For this review, take the finished solid that the model builds, in its own axes (mm). Coordinates: 2 decimals unless noted, no trailing zeros. Order: outer loops, then holes, each group sorted by start corner. A loop starts at its lowest first (then second) coordinate and runs counter-clockwise, first axis right, second up.
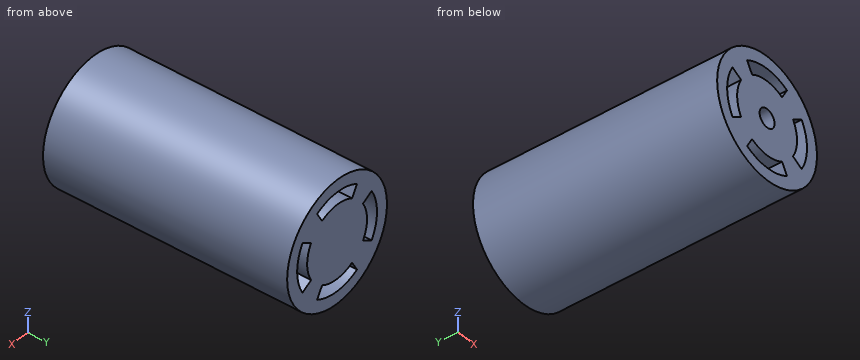
from build123d import *

# Parameters (mm, degrees)
SKETCH1_R           = 5
BOSS_EXTRUDE1_DEPTH = 20
SKETCH2_R           = 0.75
CUT_EXTRUDE1_DEPTH  = 15


with BuildPart() as part:
    # Sketch1 → Boss-Extrude1 (new body)
    with BuildSketch(Plane(origin=(0, 0, 0), x_dir=(1, 0, 0), z_dir=(0, 1, 0))):
        with Locations(Location((0, 0, 0), (0, 0, 270))):
            Circle(SKETCH1_R)
        with BuildLine():
            Line((-2, 3.464101615), (-1.5, 2.598076211))
            ThreePointArc((-1.5, 2.598076211), (0, 3), (1.5, 2.598076211))
            Line((1.5, 2.598076211), (2, 3.464101615))
            ThreePointArc((2, 3.464101615), (0, 4), (-2, 3.464101615))
        make_face(mode=Mode.SUBTRACT)
        with BuildLine():
            Line((2.598076211, -1.5), (3.464101615, -2))
            ThreePointArc((3.464101615, -2), (4, 0), (3.464101615, 2))
            Line((3.464101615, 2), (2.598076211, 1.5))
            ThreePointArc((2.598076211, 1.5), (3, 0), (2.598076211, -1.5))
        make_face(mode=Mode.SUBTRACT)
        with BuildLine():
            Line((-1.5, -2.598076211), (-2, -3.464101615))
            ThreePointArc((-2, -3.464101615), (0, -4), (2, -3.464101615))
            Line((2, -3.464101615), (1.5, -2.598076211))
            ThreePointArc((1.5, -2.598076211), (0, -3), (-1.5, -2.598076211))
        make_face(mode=Mode.SUBTRACT)
        with BuildLine():
            Line((-2.598076211, 1.5), (-3.464101615, 2))
            ThreePointArc((-3.464101615, 2), (-4, 0), (-3.464101615, -2))
            Line((-3.464101615, -2), (-2.598076211, -1.5))
            ThreePointArc((-2.598076211, -1.5), (-3, 0), (-2.598076211, 1.5))
        make_face(mode=Mode.SUBTRACT)
    extrude(amount=BOSS_EXTRUDE1_DEPTH)

    # Sketch2 → Cut-Extrude1 (cut)
    with BuildSketch(Plane.XZ):
        with Locations(Location((0, 0, 0), (0, 0, 270))):
            Circle(SKETCH2_R)
    extrude(amount=-CUT_EXTRUDE1_DEPTH, mode=Mode.SUBTRACT)


solid = part.part
1. Take a section at A-A, the plane x = 0. Give the boundary of the cut face in (y, z), plus the area to 4 significant figures.
Answer below:
outline: (0, -5) - (20, -5) - (20, -4) - (0, -4) - close; (0, -3) - (20, -3) - (20, 3) - (0, 3) - (0, 0.75) - (15, 0.75) - (15, -0.75) - (0, -0.75) - close; (0, 4) - (20, 4) - (20, 5) - (0, 5) - close
area: 137.5 mm2
2. To check wall thickness, follow L1, parallel to X at y = 5.25, z = 0; L2, parallel to X at y = 1.5, z = -2.75; L3, parallel to Z at x = -1.75, y = 18. State the ranges of each line that lie inside material, in increasing order.
Answer below:
L1: x = -5 to -4, -3 to -0.75, 0.75 to 3, 4 to 5
L2: x = -4.18 to -1.59, -1.2 to 1.2, 1.59 to 4.18
L3: z = -4.68 to -3.6, -3.03 to 3.03, 3.6 to 4.68
3. Take a section at D-D, the plane y = 18. Give the boundary of the cut face in (x, z).
Answer below:
outline: circle Ø10 at (0, 0); hole (-3.46, -2) - (-2.6, -1.5) arc R3 cw to (-2.6, 1.5) - (-3.46, 2) arc R4 ccw to start; hole (-2, -3.46) arc R4 ccw to (2, -3.46) - (1.5, -2.6) arc R3 cw to (-1.5, -2.6) - close; hole (-2, 3.46) - (-1.5, 2.6) arc R3 cw to (1.5, 2.6) - (2, 3.46) arc R4 ccw to start; hole (2.6, -1.5) - (3.46, -2) arc R4 ccw to (3.46, 2) - (2.6, 1.5) arc R3 cw to start
4. Clearance check with flat-ended pins moving along their axes: pin 1 Ø1 at (x, y) = (3, 4.5) entering from -Z; pin 2 Ø3 at (y, z) = (6.5, -3) entering from -X. State where each tip first meets the part, or that it passes through.
Answer below:
pin 1: stops at z = -4.33
pin 2: stops at x = -4.77
5. Take a section at B-B, the plane y = 11.5. Give the boundary of the cut face in (x, z).
Answer below:
outline: circle Ø10 at (0, 0); hole (-3.46, -2) - (-2.6, -1.5) arc R3 cw to (-2.6, 1.5) - (-3.46, 2) arc R4 ccw to start; hole (-2, -3.46) arc R4 ccw to (2, -3.46) - (1.5, -2.6) arc R3 cw to (-1.5, -2.6) - close; hole (-2, 3.46) - (-1.5, 2.6) arc R3 cw to (1.5, 2.6) - (2, 3.46) arc R4 ccw to start; hole circle Ø1.5 at (0, 0); hole (2.6, -1.5) - (3.46, -2) arc R4 ccw to (3.46, 2) - (2.6, 1.5) arc R3 cw to start
6. Take a section at C-C, the plane z = 0. Give the boundary of the cut face in (x, y).
Answer below:
outline: (-5, 0) - (-4, 0) - (-4, 20) - (-5, 20) - close; (-3, 0) - (-0.75, 0) - (-0.75, 15) - (0.75, 15) - (0.75, 0) - (3, 0) - (3, 20) - (-3, 20) - close; (4, 0) - (5, 0) - (5, 20) - (4, 20) - close
